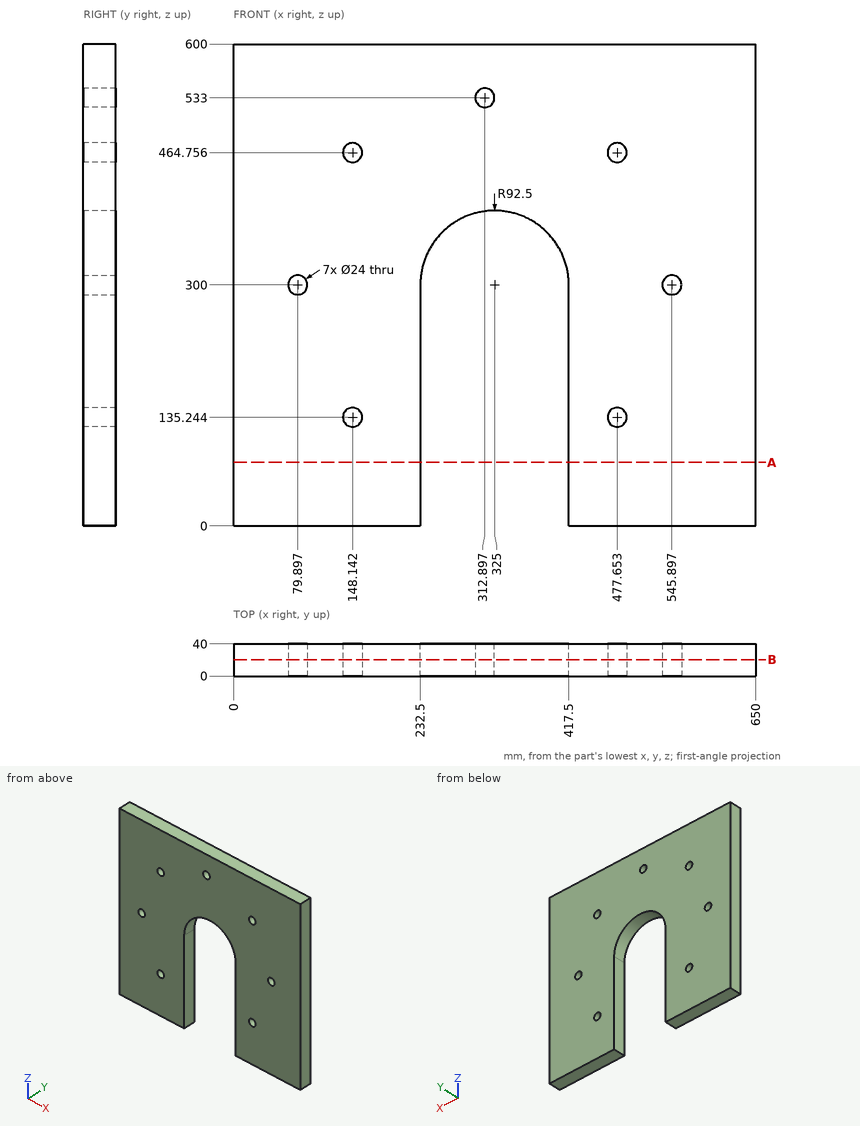
The figure shows three views and two pictorial views of one solid part (mm, origin at its lowest corner). Answer the questions. Coordinates: 2 decimals unless noted, no trailing zeros. Write each loop counter-clockwise with the first axis right and the second up, starting at its lowest first coordinate (ties: lowest second). Pieces come first, ordered by that corner, then holes. Notation, with made-up numbers: (-16.75, 17) -> (-0.75, 17) arc R23 ccw to (-0.75, 48) -> close; hole circle Ø6 at (-23.75, 28.25). An arc over 180 degrees is marked (long way). Return JSON: item names as keys, results as strings.
1. A cutting plane is placed at B-B (y = 20.5). Determine the outline of the cut face in (x, z) (1 decimal).
Found:
{"outline": "(0, 0) -> (232.5, 0) -> (232.5, 300) arc R92.5 cw to (417.5, 300) -> (417.5, 0) -> (650, 0) -> (650, 600) -> (0, 600) -> close; hole circle Ø24 at (79.9, 300); hole circle Ø24 at (148.1, 135.2); hole circle Ø24 at (148.1, 464.8); hole circle Ø24 at (312.9, 533); hole circle Ø24 at (477.7, 135.2); hole circle Ø24 at (477.7, 464.8); hole circle Ø24 at (545.9, 300)"}
2. A cutting plane is placed at A-A (z = 79). Determine the outline of the cut face in (x, y), and give its area (3 significant figures).
Found:
{"outline": "(0, 0) -> (232.5, 0) -> (232.5, 40) -> (0, 40) -> close; (417.5, 0) -> (650, 0) -> (650, 40) -> (417.5, 40) -> close", "area": "18,600 mm2"}
3. This flat-tipped pin is pushed along its axis until it touches: P1, Ø1, axis at x = 404, y = 12, coming from the -Z side (1 decimal). Where does it stop, or does it pass through?
Found:
{"P1": "z = 347.3"}
4. Find the intervals of material crossed by line 1 along X through (y, z) = (31, 136) (1 decimal); line 2 along X through (y, z) = (32, 298.5); line 3 along X through (y, z) = (28, 37.5), in increasing order. Write a range as from..to.
Found:
{"line 1": "0..136.2, 160.1..232.5, 417.5..465.7, 489.6..650", "line 2": "0..67.99, 91.8..232.5, 417.5..533.99, 557.8..650", "line 3": "0..232.5, 417.5..650"}
